from build123d import *

# Parameters (mm, degrees)
BOSS_EXTRUDE1_DEPTH = 25
CUT_EXTRUDE2_DEPTH  = 26
BOSS_EXTRUDE2_DEPTH = 0.4


with BuildPart() as part:
    # Sketch1 → Boss-Extrude1 (new body)
    with BuildSketch(Plane(origin=(0, 0, 0), x_dir=(1, 0, 0), z_dir=(0, 1, 0))):
        with BuildLine():
            ThreePointArc((1.451818925, -34.068556857), (1.641248992, -34.346908706), (1.964225605, -34.442038138))
            ThreePointArc((1.964225605, -34.442038138), (26.591847487, -21.978073076), (34.198225299, 4.555174015))
            ThreePointArc((34.198225299, 4.555174015), (23.590291339, 25.176355888), (2.324135821, 34.423627607))
            ThreePointArc((2.324135821, 34.423627607), (1.751838249, 34.289058819), (1.354061739, 33.856153382))
            ThreePointArc((1.354061739, 33.856153382), (0, 33.001534515), (-1.354061739, 33.856153382))
            ThreePointArc((-1.354061739, 33.856153382), (-1.751838249, 34.289058819), (-2.324135821, 34.423627607))
            ThreePointArc((-2.324135821, 34.423627607), (-23.590291339, 25.176355888), (-34.198225299, 4.555174015))
            ThreePointArc((-34.198225299, 4.555174015), (-26.591847487, -21.978073076), (-1.964225605, -34.442038138))
            ThreePointArc((-1.964225605, -34.442038138), (-1.641248992, -34.346908706), (-1.451818925, -34.068556857))
            ThreePointArc((-1.451818925, -34.068556857), (0, -32.945679925), (1.451818925, -34.068556857))
        make_face()
        with BuildLine():
            Line((-2.417, 3.787737139), (0, 3.787737139))
            Line((0, 3.787737139), (2.417, 3.787737139))
            ThreePointArc((2.417, 3.787737139), (0, -4.489512172), (-2.417, 3.787737139))
        make_face(mode=Mode.SUBTRACT)
    extrude(amount=BOSS_EXTRUDE1_DEPTH)

    # Sketch2 → Cut-Extrude2 (cut, through all)
    with BuildSketch(Plane(origin=(0, 0, 0), x_dir=(1, 0, 0), z_dir=(0, 1, 0))):
        with BuildLine():
            ThreePointArc((-29.852678571, -2.96944138), (-21.213203436, -21.213203436), (-2.96944138, -29.852678571))
            ThreePointArc((-2.96944138, -29.852678571), (-1.979132422, -29.698851682), (-1.187776552, -29.083928571))
            ThreePointArc((-1.187776552, -29.083928571), (0, -28.5), (1.187776552, -29.083928571))
            ThreePointArc((1.187776552, -29.083928571), (1.979132422, -29.698851682), (2.96944138, -29.852678571))
            ThreePointArc((2.96944138, -29.852678571), (21.213203436, -21.213203436), (29.852678571, -2.96944138))
            ThreePointArc((29.852678571, -2.96944138), (29.698851682, -1.979132422), (29.083928571, -1.187776552))
            ThreePointArc((29.083928571, -1.187776552), (28.5, 0), (29.083928571, 1.187776552))
            ThreePointArc((29.083928571, 1.187776552), (29.698851682, 1.979132422), (29.852678571, 2.96944138))
            ThreePointArc((29.852678571, 2.96944138), (21.213203436, 21.213203436), (2.96944138, 29.852678571))
            ThreePointArc((2.96944138, 29.852678571), (1.979132422, 29.698851682), (1.187776552, 29.083928571))
            ThreePointArc((1.187776552, 29.083928571), (0, 28.5), (-1.187776552, 29.083928571))
            ThreePointArc((-1.187776552, 29.083928571), (-1.979132422, 29.698851682), (-2.96944138, 29.852678571))
            ThreePointArc((-2.96944138, 29.852678571), (-21.213203436, 21.213203436), (-29.852678571, 2.96944138))
            ThreePointArc((-29.852678571, 2.96944138), (-29.698851682, 1.979132422), (-29.083928571, 1.187776552))
            ThreePointArc((-29.083928571, 1.187776552), (-28.5, 0), (-29.083928571, -1.187776552))
            ThreePointArc((-29.083928571, -1.187776552), (-29.698851682, -1.979132422), (-29.852678571, -2.96944138))
        make_face()
    extrude(amount=CUT_EXTRUDE2_DEPTH, mode=Mode.SUBTRACT)

    # Sketch2<2> → Boss-Extrude2 (add)
    with BuildSketch(Plane(origin=(0, 0, 0), x_dir=(1, 0, 0), z_dir=(0, 1, 0))):
        with BuildLine():
            ThreePointArc((-29.852678571, -2.96944138), (-21.213203436, -21.213203436), (-2.96944138, -29.852678571))
            ThreePointArc((-2.96944138, -29.852678571), (-1.979132422, -29.698851682), (-1.187776552, -29.083928571))
            ThreePointArc((-1.187776552, -29.083928571), (0, -28.5), (1.187776552, -29.083928571))
            ThreePointArc((1.187776552, -29.083928571), (1.979132422, -29.698851682), (2.96944138, -29.852678571))
            ThreePointArc((2.96944138, -29.852678571), (21.213203436, -21.213203436), (29.852678571, -2.96944138))
            ThreePointArc((29.852678571, -2.96944138), (29.698851682, -1.979132422), (29.083928571, -1.187776552))
            ThreePointArc((29.083928571, -1.187776552), (28.5, 0), (29.083928571, 1.187776552))
            ThreePointArc((29.083928571, 1.187776552), (29.698851682, 1.979132422), (29.852678571, 2.96944138))
            ThreePointArc((29.852678571, 2.96944138), (21.213203436, 21.213203436), (2.96944138, 29.852678571))
            ThreePointArc((2.96944138, 29.852678571), (1.979132422, 29.698851682), (1.187776552, 29.083928571))
            ThreePointArc((1.187776552, 29.083928571), (0, 28.5), (-1.187776552, 29.083928571))
            ThreePointArc((-1.187776552, 29.083928571), (-1.979132422, 29.698851682), (-2.96944138, 29.852678571))
            ThreePointArc((-2.96944138, 29.852678571), (-21.213203436, 21.213203436), (-29.852678571, 2.96944138))
            ThreePointArc((-29.852678571, 2.96944138), (-29.698851682, 1.979132422), (-29.083928571, 1.187776552))
            ThreePointArc((-29.083928571, 1.187776552), (-28.5, 0), (-29.083928571, -1.187776552))
            ThreePointArc((-29.083928571, -1.187776552), (-29.698851682, -1.979132422), (-29.852678571, -2.96944138))
        make_face()
    extrude(amount=BOSS_EXTRUDE2_DEPTH)


solid = part.part
Geometry: final body of the model. Coordinates: model frame, mm. A direction names the side the tool comes from. Coordinates: 2 decimals unless noted, no trailing zeros. Loops run counter-clockwise (first coordinate to the right, second up) from the corner with the lowest first, then second, coordinate; pieces in that order, holes last. Notation, with made-up numbers: (61, 44.25) - (89, 44.25) arc R26 cw to (89, 61.25) - close; hole circle Ø11 at (-12.5, -12.75). An arc over 180 degrees is marked (long way). Put each result on its own line as item: value. Start each with the question number.
Q1. Pin query (flat end, axial travel): pin 1 Ø6 at (y, z) = (18, -24) entering from -X; pin 2 Ø12 at (y, z) = (16.5, 13.5) entering from +X; pin 3 Ø6 at (y, z) = (3.5, 25) entering from -X. Return the tip coordinate at first contact, or that it passes through.
Q2. Pull-direction query (Z, two-part tool) for faces 3 (the cylindrical face through (0, 12, -33)), 4 (the cylindrical face through (-0.028, 12.325, 32.946)), 5 (the cylindrical face through (-21.008, 12.528, -21.416)); classes: released by +Z, released by -Z, zero draft, split by the parting line, or undercut.
Q3. Line query: line 1 (Y direction, x = 10, z = -18); line 2 (X direction, y = 2.25, z = -20); line 3 (X direction, y = 21.75, z = 8). Output: solid intervals per line, ascending.
Q4. Cut plane A-A, the plane y = 12.5. Return loops of the section in (x, z), and give its area (3 significant figures).
Q5. Cut plane B-B, the plane z = 23. Return loops of the section in (x, y).
Q6. Cut plane C-C, the plane x = -8. Return loops of the section in (y, z).
Q7. Set-up query: faces 1 (the flat face through (0, 25, 30)), 2 (the cylindrical face through (-21.416, 12.528, 21.008)). Return all of +Z, -Z, +X, -X, +Y, -Y with unobstructed straight access to the full face (end or side cutting, diameter ignored); none if empty.
Filled sheet:
1. pin 1: x = -27.37
1. pin 2: x = 33.67
1. pin 3: x = -26.57
2. face 3: released by -Z
2. face 4: released by +Z
2. face 5: undercut
3. line 1: 0 to 0.4
3. line 2: -28.11 to -22.36, 22.36 to 28.11
3. line 3: -33.56 to -28.91, 28.91 to 33.56
4. outline: (-2.32, -34.42) arc R1 ccw to (-1.35, -33.86) arc R1.5 cw to (1.35, -33.86) arc R1 ccw to (2.32, -34.42) arc R34.5 ccw to (1.96, 34.44) arc R0.5 ccw to (1.45, 34.07) arc R1.5 cw to (-1.45, 34.07) arc R0.5 ccw to (-1.96, 34.44) arc R34.5 ccw to start; hole (-29.85, -2.97) arc R30 ccw to (-2.97, -29.85) arc R2 ccw to (-1.19, -29.08) arc R1.5 cw to (1.19, -29.08) arc R2 ccw to (2.97, -29.85) arc R30 ccw to (29.85, -2.97) arc R2 ccw to (29.08, -1.19) arc R1.5 cw to (29.08, 1.19) arc R2 ccw to (29.85, 2.97) arc R30 ccw to (2.97, 29.85) arc R2 ccw to (1.19, 29.08) arc R1.5 cw to (-1.19, 29.08) arc R2 ccw to (-2.97, 29.85) arc R30 ccw to (-29.85, 2.97) arc R2 ccw to (-29.08, 1.19) arc R1.5 cw to (-29.08, -1.19) arc R2 ccw to start
4. area: 921 mm²
5. outline: (-25.71, 0) - (25.71, 0) - (25.71, 25) - (19.26, 25) - (19.26, 0.4) - (-19.26, 0.4) - (-19.26, 25) - (-25.71, 25) - close
6. outline: (0, -33.56) - (25, -33.56) - (25, -28.91) - (0.4, -28.91) - (0.4, 28.91) - (25, 28.91) - (25, 33.56) - (0, 33.56) - close
7. face 1: +Z, -Z, +X, -X, +Y
7. face 2: +Y
